Input: part model. Units: mm. Frame: model coordinates. A direction names the side the tool comes from. Give positions to 0.01 mm unless a question says otherwise; leave off trailing zeros. Write each loop counter-clockwise with the first axis right and the second up, starting at its lowest first coordinate (ties: lowest second). Pieces come first, ordered by that corner, then holes. Notation, with made-up numbers: (14, 70) - (55, 70) arc R13 cw to (55, 77) - close; hole circle Ø11 at (12.5, 52.5). An arc over 180 degrees is marked (long way). Use a Markdown table: item, result. Add a question column.
1. Section query C-C, the plane z = -19.05. Return loops of the section in (x, y), plus the area to 3 significant figures.
2. Section query D-D, the plane x = -53.34. Return loops of the section in (y, z) (1 decimal), plus the area to 3 significant figures.
3. Mould query, pull axis Z, two halves, no side actions, for faces 4 (the flat face through (0, 1, -19)), 5 (the cylindrical face through (-29.17, 16.51, -19.22)), 6 (the flat face through (-39, 1, -20.363)). Classes: released by +Z, released by -Z, zero draft, split by the parting line, or undercut.
4. Section query B-B, the plane y = 11.25. Return loops of the section in (x, z).
5. Material intervals for probe 1 along X at (y, z) = (1, -5.08) (3 decimals); probe 2 along Y at (x, z) = (-36, -8); probe 3 along X at (y, z) = (2.5, -17.5), sorted ascending.
6. Section query A-A, the plane z = -33.02. Return loops of the section in (x, y) (1 decimal), plus the area to 3 significant figures.
7. Set-up query: faces 1 (the flat face through (-33.452, 1, -24)), 2 (the cylindrical face through (-29.17, 6.458, -24.916)), 3 (the flat face through (-26.352, 2, -20)). Return all of +Z, -Z, +X, -X, +Y, -Y with unobstructed straight access to the full face (end or side cutting, diameter ignored); none if empty.
8. Pin query (flat end, axial travel): pin 1 (1.3 mm diameter, centred on x = -18, y = 0.5, fed in from +Z); pin 2 (6 mm diameter, centred on x = -46, z = -15.5, fed in from +Y); pin 3 (3 mm diameter, centred on y = 6, z = -9, fed in from +X); pin 4 (1 mm diameter, centred on y = 6, z = -13, fed in from -X). Return the tip coordinate at first contact, or that it passes through.
```python
from build123d import *

# Parameters (mm, degrees)
SKETCH1_W            = 58.42
SKETCH1_H            = 38.1
BOSS_EXTRUDE1_DEPTH  = 1.5875
BOSS_EXTRUDE2_DEPTH  = 2.8575
SKETCH4_R            = 6.35
CUT_EXTRUDE1_DEPTH   = 53.464413236
CUT_EXTRUDE2_DEPTH   = 72.324521774
MIRROR4_COPY_1_DEPTH = 72.324521774
SKETCH6_R            = 3.175
CUT_EXTRUDE3_DEPTH   = 72.324521774


with BuildPart() as part:
    # Sketch1 → Boss-Extrude1 (new body)
    with BuildSketch(Plane(origin=(0, 0, 0), x_dir=(1, 0, 0), z_dir=(0, 1, 0))):
        with Locations((-29.21, 19.05)):
            Rectangle(SKETCH1_W, SKETCH1_H)
    extrude(amount=BOSS_EXTRUDE1_DEPTH)

    # Sketch2 → Boss-Extrude2 (add, symmetric)
    with BuildSketch(Plane(origin=(-29.21, 0, 0), x_dir=(0, 0, -1), z_dir=(1, 0, 0))):
        with BuildLine():
            Line((11.43, 8.89), (11.43, 0))
            Line((11.43, 0), (26.67, 0))
            Line((26.67, 0), (26.67, 8.89))
            ThreePointArc((26.67, 8.89), (19.05, 16.51), (11.43, 8.89))
        make_face()
    extrude(amount=BOSS_EXTRUDE2_DEPTH, both=True)

    # Sketch4 → Cut-Extrude1 (cut, through all)
    with BuildSketch(Plane(origin=(-26.3525, 0, 0), x_dir=(0, 0, -1), z_dir=(1, 0, 0))):
        with Locations((19.05, 8.89)):
            Circle(SKETCH4_R)
    extrude(amount=-CUT_EXTRUDE1_DEPTH, mode=Mode.SUBTRACT)

    # Sketch5 → Cut-Extrude2 (cut, through all)
    with BuildSketch(Plane(origin=(0, 1.5875, 0), x_dir=(1, 0, 0), z_dir=(0, 1, 0))):
        Polygon((-54.61, 27.94), (-54.61, 20.363487121), (-47.840801185, 27.94), align=None)
        Polygon((-45.300801185, 27.94), (-52.07, 20.363487121), (-45.300801185, 20.363487121), align=None)
        Polygon((-42.760801185, 20.363487121), (-42.760801185, 27.94), (-35.99160237, 20.363487121), align=None)
        Polygon((-40.220801185, 27.94), (-33.45160237, 20.363487121), (-33.45160237, 27.94), align=None)
    cut_extrude2 = extrude(amount=-CUT_EXTRUDE2_DEPTH, mode=Mode.SUBTRACT)

    # Mirror2: Cut-Extrude2 across plane
    add(cut_extrude2.mirror(Plane(origin=(0, 0, -19.05), x_dir=(1, 0, 0), z_dir=(0, 0, -1))), mode=Mode.SUBTRACT)

    # Mirror3: Cut-Extrude2 across plane
    add(cut_extrude2.mirror(Plane(origin=(-29.21, 0, 0), x_dir=(0, 0, 1), z_dir=(1, 0, 0))), mode=Mode.SUBTRACT)

    # Mirror4 copy 1 sketch → Mirror4 copy 1 (cut, through all)
    with BuildSketch(Plane(origin=(-58.42, 1.5875, -38.1), x_dir=(-1, 0, 0), z_dir=(0, 1, 0))):
        Polygon((-54.61, 27.94), (-54.61, 20.363487121), (-47.840801185, 27.94), align=None)
        Polygon((-45.300801185, 27.94), (-52.07, 20.363487121), (-45.300801185, 20.363487121), align=None)
        Polygon((-42.760801185, 20.363487121), (-42.760801185, 27.94), (-35.99160237, 20.363487121), align=None)
        Polygon((-40.220801185, 27.94), (-33.45160237, 20.363487121), (-33.45160237, 27.94), align=None)
    extrude(amount=-MIRROR4_COPY_1_DEPTH, mode=Mode.SUBTRACT)

    # Sketch6 → Cut-Extrude3 (cut, through all)
    with BuildSketch(Plane(origin=(0, 1.5875, 0), x_dir=(1, 0, 0), z_dir=(0, 1, 0))):
        with Locations(Location((-53.34, 33.02, 0), (0, 0, 270))):
            Circle(SKETCH6_R)
        with Locations(Location((-5.08, 33.02, 0), (0, 0, 270))):
            Circle(SKETCH6_R)
        with Locations(Location((-5.08, 5.08, 0), (0, 0, 270))):
            Circle(SKETCH6_R)
        with Locations(Location((-53.34, 5.08, 0), (0, 0, 270))):
            Circle(SKETCH6_R)
    extrude(amount=-CUT_EXTRUDE3_DEPTH, mode=Mode.SUBTRACT)


solid = part.part
```
Result sheet:
| question | item | result |
|---|---|---|
| 1 | outline | (-58.42, 0) - (0, 0) - (0, 1.59) - (-26.35, 1.59) - (-26.35, 2.54) - (-32.07, 2.54) - (-32.07, 1.59) - (-58.42, 1.59) - close; (-32.07, 15.24) - (-26.35, 15.24) - (-26.35, 16.51) - (-32.07, 16.51) - close |
| 1 | area | 105 mm² |
| 2 | outline | (0, -38.1) - (1.6, -38.1) - (1.6, -36.2) - (0, -36.2) - close; (0, -29.8) - (1.6, -29.8) - (1.6, -27.9) - (0, -27.9) - close; (0, -21.8) - (1.6, -21.8) - (1.6, -16.3) - (0, -16.3) - close; (0, -10.2) - (1.6, -10.2) - (1.6, -8.3) - (0, -8.3) - close; (0, -1.9) - (1.6, -1.9) - (1.6, 0) - (0, 0) - close |
| 2 | area | 20.8 mm² |
| 3 | face 4 | zero draft |
| 3 | face 5 | split by the parting line |
| 3 | face 6 | undercut |
| 4 | outline | (-32.07, -26.3) - (-26.35, -26.3) - (-26.35, -24.95) - (-32.07, -24.95) - close; (-32.07, -13.15) - (-26.35, -13.15) - (-26.35, -11.8) - (-32.07, -11.8) - close |
| 5 | probe 1 | x = -58.42 to -56.515, -50.165 to -8.255, -1.905 to 0 |
| 5 | probe 2 | y = 0 to 1.59 |
| 5 | probe 3 | x = -32.07 to -26.35 |
| 6 | outline | (-58.4, 0) - (-56.5, 0) - (-56.5, 1.6) - (-58.4, 1.6) - close; (-50.2, 0) - (-8.3, 0) - (-8.3, 1.6) - (-50.2, 1.6) - close; (-1.9, 0) - (0, 0) - (0, 1.6) - (-1.9, 1.6) - close |
| 6 | area | 72.6 mm² |
| 7 | face 1 | +Y, -Y |
| 7 | face 2 | +X, -X |
| 7 | face 3 | +Z, -Z, +X, +Y |
| 8 | pin 1 | stops at z = 0 |
| 8 | pin 2 | stops at y = 1.59 |
| 8 | pin 3 | passes through |
| 8 | pin 4 | stops at x = -32.07 |
